The drawing under review shows one solid part. Ordinate dimensions are in mm from its lowest x, y, z. A direction names the side the tool comes from. Give positions to 0.01 mm unless a question says otherwise; leave off trailing zeros. Write each loop counter-clockwise with the first axis right and the second up, starting at its lowest first coordinate (ties: lowest second). Pieces come first, ordered by that corner, then holes. Notation, with made-up numbers: (8.25, 34) - (53.25, 34) arc R12 cw to (53.25, 44) - close; hole circle Ø11 at (-40, -10.75). An arc over 180 degrees is marked (long way). Write item = value, one per line.
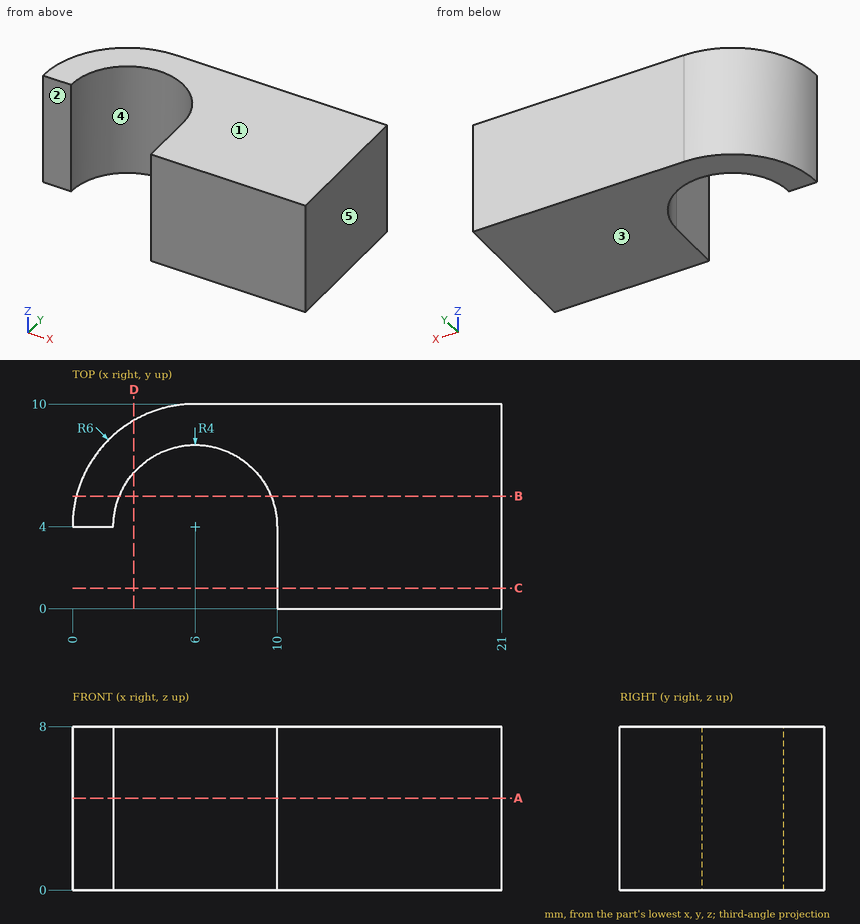
1. Take a section at D-D on x = 3. Give the boundary of the cut face in (y, z).
Findings below:
outline = (6.65, 0) - (9.2, 0) - (9.2, 8) - (6.65, 8) - close
2. Take a section at B-B on y = 5.5. Give the boundary of the cut face in (x, z).
Findings below:
outline = (0.19, 0) - (2.29, 0) - (2.29, 8) - (0.19, 8) - close; (9.71, 0) - (21, 0) - (21, 8) - (9.71, 8) - close
3. Insertion check: P1, Ø2, axis at x = 1, z = 4.5, coming from the -Y side; P2, Ø3, axis at y = 1.5, z = 4.5, coming from the -X side. Each pin has a flat end and moves straight along its axis. Give the tip position at first contact, or say it passes through.
Findings below:
P1 = 4
P2 = 10
4. For line 1 (X direction, y = 2.25, z = 1.25); line 2 (X direction, y = 4.5, z = 7.25); line 3 (X direction, y = 5.25, z = 4.75), list the stretches that pass through material, from the lowest coordinate up. Write a range as from..to.
Findings below:
line_1 = 10..21
line_2 = 0.02..2.03, 9.97..21
line_3 = 0.13..2.2, 9.8..21
5. Take a section at A-A on z = 4.5. Give the boundary of the cut face in (x, y).
Findings below:
outline = (0, 4) - (2, 4) arc R4 cw to (10, 4) - (10, 0) - (21, 0) - (21, 10) - (6, 10) arc R6 ccw to start
6. Machinability: for the marked faces 1 and 2, which of the approach directions +Z, -Z, +X, -X, +Y, -Y give a long, thin tool a straight path to every point of the face, cutting with its end or side? Answer none if there is none.
Findings below:
face_1 = +Z, +X, -X, +Y, -Y
face_2 = +Z, -Z, -X, -Y
7. Draft analysis for pull direction X (two halves, no side actions). For the marked faces 3, 4 and 5, state which applies: +X half, -X half, draft (parallel to the pull), parting line (faces both ways), or undercut.
Findings below:
face_3 = draft
face_4 = undercut
face_5 = +X half
8. Take a section at C-C on y = 1. Give the boundary of the cut face in (x, z), and give its area (3 significant figures).
Findings below:
outline = (10, 0) - (21, 0) - (21, 8) - (10, 8) - close
area = 88.0 mm²
